The listing builds one solid part. Answer for the finished solid, in the listing's coordinates (mm). Face numbers are marked on the shaded views. A direction names the side the tool comes from. Round coordinates to 2 decimals unless told otherwise and drop trailing zeros. Write each loop counter-clockwise with the first axis right and the second up, starting at its lowest first coordinate (ties: lowest second). Pieces come first, ordered by that corner, then holes.
Item 1: Find section D-D on x = 0. Give the vertices of the cut face in (y, z).
Item 2: Each of these flat-tipped pins is pushed along its axis until it touches: pin 1 (4 mm diameter, centred on x = -15.5, y = 15.5, fed in from -Z); pin 2 (4 mm diameter, centred on x = -15.5, y = -15.5, fed in from +Z); pin 3 (1.5 mm diameter, centred on x = -3.5, z = 53, fed in from -Y); pin 4 (8 mm diameter, centred on x = -4, z = 55.5, fed in from +Y). Where does it stop, or does it pass through?
Item 3: Find the intervals of material crossed by probe 1 along Y at (x, z) = (15.5, 17.5); probe 2 along Y at (x, z) = (15, 15), in increasing order.
Item 4: Find section C-C on z = 36. Give the vertices of the cut face in (x, y).
Item 5: A tool of negligible diameter and unlimited length cuts with its end or side. For the marked faces 1 and 2, from which of +Z, -Z, +X, -X, +Y, -Y can it reach the whole face along a straight path? Write none if from no direction.
Item 6: Find section A-A on x = -15.5. Give the vertices of the cut face in (y, z), then the cut area to 3 significant figures.
```python
from build123d import *

# Parameters (mm, degrees)
SKETCH1_W           = 40
SKETCH1_H           = 40
BOSS_EXTRUDE1_DEPTH = 40
SKETCH2_R           = 11
BOSS_EXTRUDE2_DEPTH = 2
SKETCH3_R           = 2.5
BOSS_EXTRUDE3_DEPTH = 20
SKETCH4_R           = 1.5
CUT_EXTRUDE1_DEPTH  = 49.989794856
SKETCH4_3_R         = 1.5
CUT_EXTRUDE2_DEPTH  = 49.989794856


with BuildPart() as part:
    # Sketch1 → Boss-Extrude1 (new body)
    with BuildSketch(Plane.XY):
        Rectangle(SKETCH1_W, SKETCH1_H)
    extrude(amount=BOSS_EXTRUDE1_DEPTH)

    # Sketch2 → Boss-Extrude2 (add)
    with BuildSketch(Plane.XY.offset(40)):
        Circle(SKETCH2_R)
    extrude(amount=BOSS_EXTRUDE2_DEPTH)

    # Sketch3 → Boss-Extrude3 (add)
    with BuildSketch(Plane.XY.offset(42)):
        Circle(SKETCH3_R)
    extrude(amount=BOSS_EXTRUDE3_DEPTH)

    # Sketch4 → Cut-Extrude1 (cut, through all)
    with BuildSketch(Plane.XY.offset(40)):
        with Locations((-15.5, 15.5)):
            Circle(SKETCH4_R)
        with Locations(Location((-15.5, -15.5, 0), (0, 0, 180))):
            Circle(SKETCH4_R)
        with Locations(Location((15.5, 15.5, 0), (0, 0, 180))):
            Circle(SKETCH4_R)
    extrude(amount=-CUT_EXTRUDE1_DEPTH, mode=Mode.SUBTRACT)

    # Sketch4_3 → Cut-Extrude2 (cut, through all)
    with BuildSketch(Plane.XY.offset(40)):
        with Locations((-15.5, 15.5)):
            Circle(SKETCH4_3_R)
        with Locations(Location((-15.5, -15.5, 0), (0, 0, 180))):
            Circle(SKETCH4_3_R)
        with Locations((15.5, -15.5)):
            Circle(SKETCH4_3_R)
        with Locations(Location((15.5, 15.5, 0), (0, 0, 180))):
            Circle(SKETCH4_3_R)
    extrude(amount=-CUT_EXTRUDE2_DEPTH, mode=Mode.SUBTRACT)


solid = part.part
```
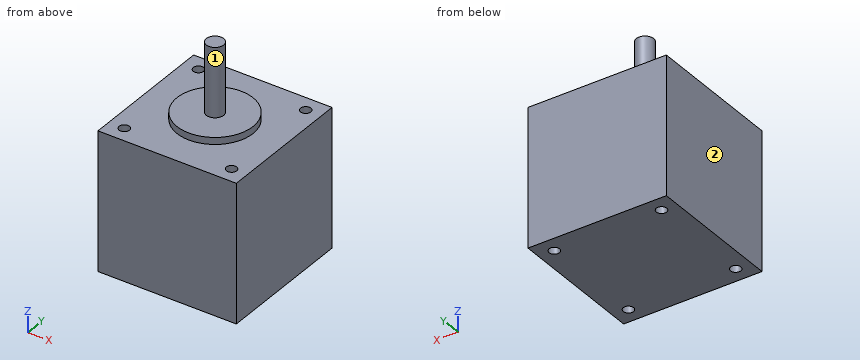
Check values:
1. outline: (-20, 0) - (20, 0) - (20, 40) - (11, 40) - (11, 42) - (2.5, 42) - (2.5, 62) - (-2.5, 62) - (-2.5, 42) - (-11, 42) - (-11, 40) - (-20, 40) - close
2. pin 1: stops at z = 0
2. pin 2: stops at z = 40
2. pin 3: passes through
2. pin 4: stops at y = 2.5
3. probe 1: y = -20 to -17, -14 to 14, 17 to 20
3. probe 2: y = -20 to -16.91, -14.09 to 14.09, 16.91 to 20
4. outline: (-20, -20) - (20, -20) - (20, 20) - (-20, 20) - close; hole circle Ø3 at (-15.5, -15.5); hole circle Ø3 at (-15.5, 15.5); hole circle Ø3 at (15.5, -15.5); hole circle Ø3 at (15.5, 15.5)
5. face 1: +Z
5. face 2: +Z, -Z, -X, +Y, -Y
6. outline: (-20, 0) - (-17, 0) - (-17, 40) - (-20, 40) - close; (-14, 0) - (14, 0) - (14, 40) - (-14, 40) - close; (17, 0) - (20, 0) - (20, 40) - (17, 40) - close
6. area: 1,360 mm2
